Could you check a few things on this model? Use its own coordinates, in mm. A direction names the side the tool comes from. Coordinates: 2 decimals unless noted, no trailing zeros. Loops run counter-clockwise (first coordinate to the right, second up) from the corner with the lowest first, then second, coordinate; pieces in that order, holes last. Notation, with made-up numbers: M 61.5,50.5 L 91.5,50.5 A21 ccw 91.5,57.5 Z; hole C 2.25,65 d8. An arc over 180 degrees is marked long. Use one line per item in the form item = value. Start each with the question number.
Autodesk Inventor part; units mm, degrees
ref_plane "YZ Plane" through (0, 0, 0) normal (1, 0, 0) x (0, 1, 0)
ref_plane "XZ Plane" through (0, 0, 0) normal (0, 1, 0) x (-1, 0, 0)
ref_plane "XY Plane" through (0, 0, 0) normal (0, 0, 1) x (1, 0, 0)
sketch "Sketch1" plane through (0, 0, 0) normal (0, 0, 1) x (1, 0, 0)
  line L0 (0, 0) -> (0, 40)
  line L1 (0, 0) -> (63, 0)
  line L2 (63, 0) -> (63, 5)
  line L3 (63, 5) -> (9, 5)
  arc A0 (9, 40) -> (0, 40) centre (4.5, 40) ccw
  line L4 (9, 40) -> (9, 5)
  circle A1 centre (4.5, 40) radius 2.5
  dimension "d0" = 40
  dimension "d2" = 5
  dimension "d6" = 4.5
  dimension "d7" = 5
  dimension "d8" = 9
  dimension "d9" = 54
  dimension "d47" = 32.5
extrude "Extrusion1" add sketch "Sketch1" along normal blind 20
sketch "Sketch2" plane through (9, 5, 0) normal (0, 1, 0) x (1, 0, 0)
  line L0 (0, 0) -> (0, -20)
  circle A0 centre (26, -10) radius 10
  line L1 (0, 0) -> (54, 0)
  circle A1 centre (54, -10) radius 2.8
  line L2 (54, 0) -> (54, -20)
  point P0 (-9, 0)
  dimension "d14" = 20
  dimension "d16" = 26
  dimension "d20" = 5.6
  dimension "d21" = 10
  dimension "d22" = 15.2
  dimension "d67" = 0
sketch "Sketch7" plane through (9, 5, 0) normal (1, 0, 0) x (0, 0, -1)
  line L0 (-10, 41.0364) -> (-10, 39.6436)
  line L1 (0, 39.5) -> (-20, 39.5)
  line L2 (-2.5, 39.5) -> (-2.5, 25.5)
  line L3 (-17.5, 39.5) -> (-17.5, 25.5)
  line L4 (-17.5, 39.5) -> (-2.5, 39.5)
  line L5 (0, 32.5) -> (-20, 32.5)
  line L6 (-17.5, 25.5) -> (-2.5, 25.5)
  point P0 (0, -5)
  dimension "d40" = 14
  dimension "d41" = 14
  dimension "d42" = 15
extrude "Extrusion5" cut sketch "Sketch7" against normal blind 14
extrude "Extrusion6" add sketch "Sketch2" along normal blind 25
sketch "Sketch9" plane through (35, 30, 10) normal (0, 1, 0) x (1, 0, 0)
  circle A0 centre (0, 0) radius 8
  point P0 (-35, 10)
  dimension "d50" = 16
extrude "Extrusion7" cut sketch "Sketch9" against normal blind 31
sketch "Sketch10" plane through (9, 5, 20) normal (0, 1, 0) x (1, 0, 0)
  line L0 (6, 8) -> (12, 8)
  line L1 (12, 8) -> (12, 12)
  line L2 (12, 12) -> (6, 12)
  line L3 (6, 12) -> (6, 8)
  line L4 (26, 0) -> (0, 0)
  line L5 (0, 2.5) -> (0, 17.5)
  point P0 (-9, 20)
  dimension "d53" = 6
  dimension "d54" = 4
  dimension "d55" = 8
  dimension "d56" = 6
extrude "Extrusion8" add sketch "Sketch10" along normal blind 6
sketch "Sketch11" plane through (21, 5, 8) normal (0, 0, -1) x (-1, 0, 0)
  line L0 (2, 4) -> (4, 4)
  line L1 (6, 0) -> (6, 6)
  line L2 (12, 0) -> (-14, 0)
  line L3 (0, 0) -> (6, 0)
  line L4 (0, 1.5) -> (0, 0)
  line L5 (6, 0) -> (0, 0)
  line L6 (0, 0) -> (3, 0)
  line L7 (0, 1.5) -> (2, 1.5)
  line L8 (2, 1.5) -> (2, 4)
  line L9 (3, 0) -> (0, 0)
  line L10 (4, 4) -> (4, 0)
  line L11 (0, 0) -> (6, 0)
  line L12 (0, 0) -> (4, 0)
  point P0 (21, -5)
  dimension "d59" = 2
  dimension "d60" = 2
  dimension "d61" = 4
  dimension "d62" = 1.5
extrude "Extrusion9" cut sketch "Sketch11" against normal blind 4
sketch "Sketch12" plane through (35, 5, 0) normal (0, 1, 0) x (1, 0, 0)
  line L0 (28, 0) -> (28, -20)
  arc A0 (28, -20) -> (28, 0) centre (28, -10) ccw
  line L1 (28, 0) -> (-35, 0)
  line L2 (28, 0) -> (28, -20)
extrude "Extrusion10" add sketch "Sketch12" against normal blind 5
equation "\"d21\" = d19"
equation "\"d40\" = d41"
equation "\"d19\" = 0.5 * d14"
properties part number "ValveBaseMk2.4"
Item 1: I want a section at A-A (y = 26). Write out the boundary of the cut face in (x, z).
Item 2: I want a section at D-D (y = 33). Write out the boundary of the cut face in (x, z), plus the area to 3 significant figures.
Item 3: Please list where these lines run through material, in increasing order: line 1 along Y through (x, z) = (4.5, 1.9); line 2 along X through (y, z) = (23, 8.75); line 3 along X through (y, z) = (17, 8.25).
Item 4: For faces 1 (the flat face through (18, 9.3, 8)), 2 (the cylindrical face through (32.83, 17.32, 0.24)), 3 (the flat face through (15, 8, 10)), which set-ups out of +Z, -Z, +X, -X, +Y, -Y let a thin tool reach every point of the face, with its end or its side?
Item 5: I want a section at B-B (x = 4.5). Write out the boundary of the cut face in (y, z), plus the area to 3 significant figures.
Item 6: I want a section at C-C (z = 10). Write out the boundary of the cut face in (x, y).
Item 7: I'm going to push flat-ended pins straight in: P1, Ø12, axis at y = 17.5, z = 16.5, coming from the +X side (3 decimals); P2, Ø6, axis at x = 19, z = 14, coming from the +Y side; P3, Ø1.5, axis at x = 26.5, z = 10, coming from the +Y side. Where does each tip first touch, or does it pass through?
Item 8: Thinking about a two-plate mould opening in X: for faces 4 (the cylindrical face through (4.4, 44.5, 18.7)), 5 (the flat face through (44, 0, 10)), 6 (the cylindrical face through (3.96, 42.44, 18.73)), 7 (the flat face through (0, 15, 10)), which applies, pulls with the +X half, pulls with the -X half, needs draft (parallel to the pull), parting line crosses it, or undercut?
Worked answers:
q1.outline = M 0,0 L 9,0 L 9,20 L 0,20 Z; C 35,10 d20; C 63,10 d5.6; hole C 35,10 d16
q2.outline = M 0,0 L 9,0 L 9,2.5 L 0,2.5 Z; M 0,17.5 L 9,17.5 L 9,20 L 0,20 Z
q2.area = 45.0 mm²
q3.line_1 = 0 to 37.5, 42.5 to 44.5
q3.line_2 = 0 to 9, 25.08 to 27.1, 42.9 to 44.92, 60.49 to 65.51
q3.line_3 = 0 to 9, 25.15 to 27.19, 42.81 to 44.85, 60.81 to 65.19
q4.face_1 = -Z, +Y
q4.face_2 = +Y
q4.face_3 = +Z, -Z, +Y
q5.outline = M 0,0 L 37.5,0 L 37.5,2.5 L 30.5,2.5 L 30.5,17.5 L 37.5,17.5 L 37.5,20 L 0,20 Z; M 42.5,0 L 44.5,0 L 44.5,2.5 L 42.5,2.5 Z; M 42.5,17.5 L 44.5,17.5 L 44.5,20 L 42.5,20 Z
q5.area = 655 mm²
q6.outline = M 0,0 L 27,0 L 27,30 L 25,30 L 25,5 L 17,5 L 17,9 L 19,9 L 19,6.5 L 21,6.5 L 21,11 L 15,11 L 15,5 L 9,5 L 9,30.5 L 0,30.5 Z; M 43,0 L 73,0 L 73,5 L 65.8,5 L 65.8,30 L 60.2,30 L 60.2,5 L 45,5 L 45,30 L 43,30 Z
q7.P1 = 65.755
q7.P2 = 11
q7.P3 = 30
q8.face_4 = parting line crosses it
q8.face_5 = needs draft
q8.face_6 = undercut
q8.face_7 = pulls with the -X half
